Source: CAD feature listing. Evaluate the final solid. Frame: model axes, mm. Face numbers are marked on the shaded views. Coordinates: 2 decimals unless noted, no trailing zeros. Loops run counter-clockwise (first coordinate to the right, second up) from the corner with the lowest first, then second, coordinate; pieces in that order, holes last.
Item 1: Section query B-B, the plane y = -14.8. Return the cut outline in (x, z).
Item 2: Pin query (flat end, axial travel): pin 1 Ø3 at (x, y) = (-45, -58.2) entering from -Z; pin 2 Ø6 at (y, z) = (-59, 1) entering from -X; pin 3 Ø1.2 at (x, y) = (53, 28) entering from -Z; pin 4 Ø6 at (x, y) = (28.5, 4.5) entering from -Z. Return the tip coordinate at first contact, or that it passes through.
Item 3: Pull-direction query (X, two-part tool) for the marked faces 1 and 2; classes: +X half, -X half, draft (parallel to the pull), parting line (faces both ways), or undercut.
Item 4: Section query C-C, the plane z = -7.5. Return the cut outline in (x, y).
Item 5: Line query: probe 1 along Y at (x, z) = (52.1, -8); probe 2 along Y at (x, z) = (48.3, 1.6); probe 3 along Y at (x, z) = (53.5, -10.25). Output: solid intervals per line, ascending.
Item 6: Section query A-A, the plane x = -20. Return the cut outline in (y, z), then the cut area to 4 significant figures.
Item 7: Section query D-D, the plane y = -63. Return the cut outline in (x, z).
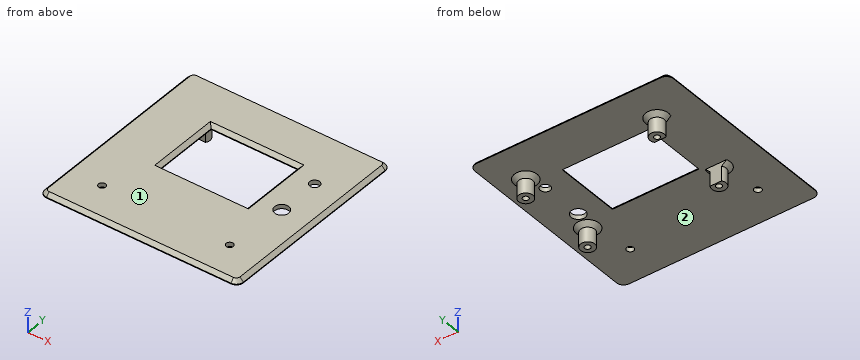
```python
from build123d import *

# Parameters (mm, degrees)
SKETCH1_W           = 140
SKETCH1_H           = 140
SKETCH1_R           = 3.5
SKETCH1_R_2         = 2
SKETCH1_R_3         = 5
SKETCH1_R_4         = 2.5
SKETCH1_W_2         = 61
SKETCH1_H_2         = 46
BOSS_EXTRUDE1_DEPTH = 3
CHAMFER1_SIZE       = 2.5
FILLET1_R           = 5
CHAMFER2_SIZE       = 2.5
SKETCH2_R           = 5
BOSS_EXTRUDE3_DEPTH = 13.3
CHAMFER3_SIZE       = 3
SKETCH4_R           = 2
CUT_EXTRUDE1_DEPTH  = 8
SKETCH6_W           = 89.583277887
SKETCH6_H           = 51
CUT_EXTRUDE2_DEPTH  = 13.3
SKETCH7_R           = 4.27453946
SKETCH7_R_2         = 4.288417291
SKETCH7_R_3         = 5.40642801
SKETCH7_R_4         = 4.2459997
BOSS_EXTRUDE4_DEPTH = 3


with BuildPart() as part:
    # Sketch1 → Boss-Extrude1 (new body)
    with BuildSketch(Plane.XY):
        with Locations((0, -13.199218639)):
            Rectangle(SKETCH1_W, SKETCH1_H)
        with Locations((48.3, 15.4)):
            Circle(SKETCH1_R, mode=Mode.SUBTRACT)
        with Locations((-40.5, 28.4)):
            Circle(SKETCH1_R_2, mode=Mode.SUBTRACT)
        with Locations((52.1, 28.4)):
            Circle(SKETCH1_R_2, mode=Mode.SUBTRACT)
        with Locations((52.1, -28.4)):
            Circle(SKETCH1_R_2, mode=Mode.SUBTRACT)
        with Locations((-40.5, -28.4)):
            Circle(SKETCH1_R_2, mode=Mode.SUBTRACT)
        with Locations((48.3, -14.8)):
            Circle(SKETCH1_R_3, mode=Mode.SUBTRACT)
        with Locations((45, -58.199218639)):
            Circle(SKETCH1_R_4, mode=Mode.SUBTRACT)
        with Locations((-45, -58.199218639)):
            Circle(SKETCH1_R_4, mode=Mode.SUBTRACT)
        Rectangle(SKETCH1_W_2, SKETCH1_H_2, mode=Mode.SUBTRACT)
    extrude(amount=BOSS_EXTRUDE1_DEPTH)

    # Chamfer1
    chamfer1_edges = [part.edges().sort_by_distance(p)[0] for p in [
        (30.5, 0, 3),
        (0, 23, 3),
        (-30.5, 0, 3),
        (0, -23, 3),
    ]]
    chamfer(chamfer1_edges, length=CHAMFER1_SIZE)

    # Fillet1
    fillet1_edges = [part.edges().sort_by_distance(p)[0] for p in [
        (70, -83.199218639, 1.5),
        (-70, -83.199218639, 1.5),
        (-70, 56.800781361, 1.5),
        (70, 56.800781361, 1.5),
    ]]
    fillet(fillet1_edges, radius=FILLET1_R)

    # Chamfer2
    chamfer2_edges = [part.edges().sort_by_distance(p)[0] for p in [
        (-70, -13.199218639, 3),
        (0, 56.800781361, 3),
        (70, -13.199218639, 3),
        (0, -83.199218639, 3),
        (-68.535533906, -81.734752545, 3),
        (68.535533906, -81.734752545, 3),
        (68.535533906, 55.336315267, 3),
        (-68.535533906, 55.336315267, 3),
    ]]
    chamfer(chamfer2_edges, length=CHAMFER2_SIZE)

    # Sketch2 → Boss-Extrude3 (add)
    with BuildSketch(Plane.XY):
        with Locations((52.1, 28.4)):
            Circle(SKETCH2_R)
        with Locations((52.1, -28.4)):
            Circle(SKETCH2_R)
        with Locations((-40.5, 28.4)):
            Circle(SKETCH2_R)
        with Locations((-40.5, -28.4)):
            Circle(SKETCH2_R)
    extrude(amount=-BOSS_EXTRUDE3_DEPTH)

    # Chamfer3
    chamfer3_edges = [part.edges().sort_by_distance(p)[0] for p in [
        (47.1, 28.4, 0),
        (47.1, -28.4, 0),
        (-45.5, 28.4, 0),
        (-45.5, -28.4, 0),
    ]]
    chamfer(chamfer3_edges, length=CHAMFER3_SIZE)

    # Sketch4 → Cut-Extrude1 (cut)
    with BuildSketch(Plane(origin=(0, 0, -13.3), x_dir=(-1, 0, 0), z_dir=(0, 0, -1))):
        with Locations((-52.1, 28.4)):
            Circle(SKETCH4_R)
        with Locations((40.5, 28.4)):
            Circle(SKETCH4_R)
        with Locations((40.5, -28.4)):
            Circle(SKETCH4_R)
        with Locations((-52.1, -28.4)):
            Circle(SKETCH4_R)
    extrude(amount=-CUT_EXTRUDE1_DEPTH, mode=Mode.SUBTRACT)

    # Sketch6 → Cut-Extrude2 (cut)
    with BuildSketch(Plane(origin=(0, 0, -13.3), x_dir=(-1, 0, 0), z_dir=(0, 0, -1))):
        with Locations((25.208361056, 0)):
            Rectangle(SKETCH6_W, SKETCH6_H)
    extrude(amount=-CUT_EXTRUDE2_DEPTH, mode=Mode.SUBTRACT)

    # Sketch7 → Boss-Extrude4 (add)
    with BuildSketch(Plane.XY.offset(3)):
        with Locations((-40.5, 28.4)):
            Circle(SKETCH7_R)
        with Locations((-40.5, -28.4)):
            Circle(SKETCH7_R_2)
        with Locations((52.1, 28.4)):
            Circle(SKETCH7_R_3)
        with Locations((52.1, -28.4)):
            Circle(SKETCH7_R_4)
    extrude(amount=-BOSS_EXTRUDE4_DEPTH)


solid = part.part
```
Verdict:
1. outline: (-70, 0) - (-30.5, 0) - (-30.5, 0.5) - (-33, 3) - (-67.5, 3) - (-70, 0.5) - close; (30.5, 0) - (43.3, 0) - (43.3, 3) - (33, 3) - (30.5, 0.5) - close; (53.3, 0) - (70, 0) - (70, 0.5) - (67.5, 3) - (53.3, 3) - close
2. pin 1: passes through
2. pin 2: stops at x = -70
2. pin 3: stops at z = -5.3
2. pin 4: stops at z = 0
3. face 1: draft
3. face 2: undercut
4. outline: (-44.57, -25.5) arc R5 ccw (long way) to (-36.43, -25.5) - close; (-44.57, 25.5) - (-36.43, 25.5) arc R5 ccw (long way) to start; circle Ø10 at (52.1, -28.4); circle Ø10 at (52.1, 28.4); hole circle Ø4 at (-40.5, -28.4); hole circle Ø4 at (-40.5, 28.4); hole circle Ø4 at (52.1, -28.4); hole circle Ø4 at (52.1, 28.4)
5. probe 1: y = -33.4 to -30.4, -26.4 to -23.4, 23.4 to 26.4, 30.4 to 33.4
5. probe 2: y = -82.1 to -19.8, -9.8 to 11.9, 18.9 to 55.7
5. probe 3: y = -33.2 to -29.83, -26.97 to -23.6, 23.6 to 26.97, 29.83 to 33.2
6. outline: (-83.2, 0) - (-23, 0) - (-23, 0.5) - (-25.5, 3) - (-80.7, 3) - (-83.2, 0.5) - close; (23, 0) - (56.8, 0) - (56.8, 0.5) - (54.3, 3) - (25.5, 3) - (23, 0.5) - close
6. area: 269.5 mm2
7. outline: (-70, 0) - (70, 0) - (70, 0.5) - (67.5, 3) - (-67.5, 3) - (-70, 0.5) - close
